```python
from build123d import *

# Parameters (mm, degrees)
SKETCH1_W           = 10
SKETCH1_H           = 8
SKETCH1_R           = 1.75
BOSS_EXTRUDE2_DEPTH = 8


with BuildPart() as part:
    # Sketch1 → Boss-Extrude2 (new body)
    with BuildSketch(Plane(origin=(0, 0, 0), x_dir=(1, 0, 0), z_dir=(0, 1, 0))):
        with BuildLine():
            Line((-92, 0), (-8, 0))
            ThreePointArc((-8, 0), (-2.343145751, 2.343145751), (0, 8))
            Line((0, 8), (0, 10))
            ThreePointArc((0, 10), (-0.292893219, 10.707106781), (-1, 11))
            Line((-1, 11), (-10, 11))
            Line((-10, 11), (-10, 19))
            Line((-10, 19), (-1, 19))
            ThreePointArc((-1, 19), (-0.292893219, 19.292893219), (0, 20))
            Line((0, 20), (0, 67))
            ThreePointArc((0, 67), (-2.343145751, 72.656854249), (-8, 75))
            Line((-8, 75), (-92, 75))
            ThreePointArc((-92, 75), (-97.656854249, 72.656854249), (-100, 67))
            Line((-100, 67), (-100, 20))
            ThreePointArc((-100, 20), (-99.707106781, 19.292893219), (-99, 19))
            Line((-99, 19), (-90, 19))
            Line((-90, 19), (-90, 11))
            Line((-90, 11), (-99, 11))
            ThreePointArc((-99, 11), (-99.707106781, 10.707106781), (-100, 10))
            Line((-100, 10), (-100, 8))
            ThreePointArc((-100, 8), (-97.656854249, 2.343145751), (-92, 0))
        make_face()
        with Locations((-85, 48)):
            Rectangle(SKETCH1_W, SKETCH1_H, mode=Mode.SUBTRACT)
        with Locations((-15, 48)):
            Rectangle(SKETCH1_W, SKETCH1_H, mode=Mode.SUBTRACT)
        with Locations((-74.74, 40)):
            Circle(SKETCH1_R, mode=Mode.SUBTRACT)
        with BuildLine():
            Line((-32.110832625, 17.868191938), (-36.353473312, 22.110832625))
            ThreePointArc((-36.353473312, 22.110832625), (-65.909902577, 55.909902577), (-32.110832625, 26.353473312))
            Line((-32.110832625, 26.353473312), (-27.868191938, 22.110832625))
            Line((-27.868191938, 22.110832625), (-32.110832625, 17.868191938))
        make_face(mode=Mode.SUBTRACT)
        with Locations((-25.26, 40)):
            Circle(SKETCH1_R, mode=Mode.SUBTRACT)
    extrude(amount=BOSS_EXTRUDE2_DEPTH)


solid = part.part
```
Here's how the part is built. I have some questions about the finished solid (model axes, mm). A direction names the side the tool comes from. Give positions to 0.01 mm unless a question says otherwise; leave off trailing zeros. Loops run counter-clockwise (first coordinate to the right, second up) from the corner with the lowest first, then second, coordinate; pieces in that order, holes last. Notation, with made-up numbers: M 22,32 L 54,32 A28 ccw 54,55 Z; hole C 15,81 d1. An arc over 180 degrees is marked long. Use one line per item in the form item = value. Start each with the question number.
Q1. If we section it at C-C (z = -34.5): Write out the boundary of the cut face in (x, y).
Q2. Which directions (+Z, -Z, +X, -X, +Y, -Y) give clear straight access to the entire face, cutting with the end or side of a thin tool? Please do faces 1 (the flat face through (-30.02, 3.94, -24.26)), 2 (the flat face through (-10, 4, -15)), 3 (the flat face through (-73, 8, -38)).
Q3. Will these pins go through, and if not, where does the flat tip stop? pin 1 Ø3 at (x, z) = (-74.74, -40) entering from +Y; pin 2 Ø4 at (x, y) = (-5.5, 2) entering from +Z.
Q4. I need wall thicknesses on line 1 along Z through (x, y) = (-50.5, 3); line 2 along Z through (x, y) = (-74.74, 6); line 3 along X through (y, z) = (4, -40). Which ranges of each line are inside material? Lowest first, please.
Q5. If we section it at A-A (x = -50): Write out the boundary of the cut face in (y, z), then the cut area to 3 significant figures.
Q6. If we section it at B-B (y = 2.5): State how many separate pieces and enclosed holes the cut face has, then the cut area to 3 significant figures.
Q7. Thinking about a two-plate mould opening in X: for faces 4 (the flat face through (-73, 0, -38)), 5 (the cylindrical face through (-2.406, 3.944, -2.281)), 6 (the cylindrical face through (-97.719, 3.944, -2.406)), 7 (the cylindrical face through (-75.12, 3.94, -38.29)), which applies, +X half, -X half, draft (parallel to the pull), parting line (faces both ways), or undercut?
Taken from the geometry:
q1.outline = M -100,0 L -71.82,0 L -71.82,8 L -100,8 Z; M -28.18,0 L 0,0 L 0,8 L -28.18,8 Z
q2.face_1 = +Y, -Y
q2.face_2 = +X, +Y, -Y
q2.face_3 = +Z, -Z, +X, -X, +Y
q3.pin_1 = through
q3.pin_2 = -0.02
q4.line_1 = -75 to -62.49, -17.51 to 0
q4.line_2 = -75 to -41.75, -38.25 to 0
q4.line_3 = -100 to -76.49, -72.99 to -72.5, -27.5 to -27.01, -23.51 to 0
q5.outline = M 0,-75 L 8,-75 L 8,-62.5 L 0,-62.5 Z; M 0,-17.5 L 8,-17.5 L 8,0 L 0,0 Z
q5.area = 240 mm^2
q6.separate_pieces = 1
q6.enclosed_holes = 5
q6.area = 5,480 mm^2
q7.face_4 = draft
q7.face_5 = +X half
q7.face_6 = -X half
q7.face_7 = undercut
